Verification items for the finished model (mm, model axes). Face numbers are marked on the shaded views. A direction names the side the tool comes from. Coordinates: 2 decimals unless noted, no trailing zeros. Order: outer loops, then holes, each group sorted by start corner. A loop starts at its lowest first (then second) coordinate and runs counter-clockwise, first axis right, second up. Notation, with made-up numbers: M 31.5,76.5 L 73.5,76.5 A17 cw 73.5,99.5 Z; hole C -2,47.5 d9. An arc over 180 degrees is marked long. Return JSON: item names as keys, results as strings. Group by question number.
Q1. Access from +Z, -Z, +X, -X, +Y, -Y to the whole of each face (thin tool, end or side, straight path). Record for the marked faces 4, 5 and 6.
Q2. Section check A-A, the plane z = 43.5. Enter the section's corners in (x, y).
Q3. Mould release check, pull along X, two halves, no side actions. Record for the marked faces 1, 2 and 3: pulls with the +X half, pulls with the -X half, needs draft (parallel to the pull), parting line crosses it, or undercut.
Q4. Thickness scan on probe 1 along X at (y, z) = (16.25, 8); probe 2 along X at (y, z) = (5, -51.5); probe 3 along Z at (x, y) = (-12, 2.5). Record the ranges inside material, lowest first.
Q5. Go/stop test with flat-tipped pins: pin 1 Ø10 at (x, y) = (4.5, 8.5) entering from -Z; pin 2 Ø10 at (y, z) = (22.5, 5) entering from -X; pin 3 Ø0.8 at (x, y) = (-26, 11) entering from +Z; pin 4 Ø1.5 at (x, z) = (-14.5, -54.5) entering from +Y. Record where each tip stops, or that it passes through.
from build123d import *

# Parameters (mm, degrees)
SKETCH2_W                                       = 55
SKETCH2_H                                       = 135
BOSS_EXTRUDE1_DEPTH                             = 27
SKETCH3_W                                       = 40
SKETCH3_H                                       = 120
CUT_EXTRUDE1_DEPTH                              = 23
SKETCH19_W                                      = 12
SKETCH19_H                                      = 10
CUT_EXTRUDE7_DEPTH                              = 55
SKETCH20_R                                      = 1.25
SKETCH20_W                                      = 9.5
SKETCH20_H                                      = 76
CUT_EXTRUDE8_DEPTH                              = 6
CHAMFER1_SIZE                                   = 10
SKETCH22_R                                      = 0.75
CUT_EXTRUDE10_DEPTH                             = 10
SKETCH23_W                                      = 21.5
SKETCH23_H                                      = 21.5
CUT_EXTRUDE11_DEPTH                             = 1.5
SKETCH24_W                                      = 16
SKETCH24_H                                      = 24
BOSS_EXTRUDE2_DEPTH                             = 7
SKETCH26_W                                      = 11
SKETCH26_H                                      = 4.5
CUT_EXTRUDE13_DEPTH                             = 24
SKETCH27_W                                      = 14.142135623
SKETCH27_H                                      = 3.5
BOSS_EXTRUDE3_DEPTH                             = 8
SKETCH31_W                                      = 29
SKETCH31_H                                      = 10
CUT_EXTRUDE17_DEPTH                             = 3
SKETCH32_W                                      = 8.142135623
SKETCH32_H                                      = 10
CUT_EXTRUDE18_DEPTH                             = 3
MIRROR8_COPY_1_SKETCH_W                         = 8.142135623
MIRROR8_COPY_1_SKETCH_H                         = 10
MIRROR8_COPY_1_DEPTH                            = 3
CSK_FOR_M3_FLAT_HEAD_MACHINE_SCREW2_D           = 3.2
CSK_FOR_M3_FLAT_HEAD_MACHINE_SCREW2_CSINK_D     = 6.3
CSK_FOR_M3_FLAT_HEAD_MACHINE_SCREW2_CSINK_ANGLE = 90
FILLET3_R                                       = 4
MIRROR14_COPY_1_SKETCH_W                        = 14.142135623
MIRROR14_COPY_1_SKETCH_H                        = 3.5
MIRROR14_COPY_1_DEPTH                           = 8
FILLET3_OF_MIRROR14_R                           = 4
FILLET4_R                                       = 4
CSK_FOR_M3_FLAT_HEAD_MACHINE_SCREW3_D           = 3.2
CSK_FOR_M3_FLAT_HEAD_MACHINE_SCREW3_CSINK_D     = 6.3
CSK_FOR_M3_FLAT_HEAD_MACHINE_SCREW3_CSINK_ANGLE = 90
SKETCH46_W                                      = 5.75
SKETCH46_H                                      = 23.5
CUT_EXTRUDE20_DEPTH                             = 2.5


with BuildPart() as part:
    # Sketch2 → Boss-Extrude1 (new body)
    with BuildSketch(Plane(origin=(0, 0, 0), x_dir=(1, 0, 0), z_dir=(0, 1, 0))):
        Rectangle(SKETCH2_W, SKETCH2_H)
    extrude(amount=BOSS_EXTRUDE1_DEPTH)

    # Sketch3 → Cut-Extrude1 (cut)
    with BuildSketch(Plane.XZ):
        Rectangle(SKETCH3_W, SKETCH3_H)
    extrude(amount=-CUT_EXTRUDE1_DEPTH, mode=Mode.SUBTRACT)

    # Sketch19 → Cut-Extrude7 (cut)
    with BuildSketch(Plane(origin=(27.5, 0, 0), x_dir=(0, 0, -1), z_dir=(1, 0, 0))):
        with Locations((-32, 16)):
            Rectangle(SKETCH19_W, SKETCH19_H)
        with Locations((-16, 16)):
            Rectangle(SKETCH19_W, SKETCH19_H)
        with Locations((0, 16)):
            Rectangle(SKETCH19_W, SKETCH19_H)
        with Locations((16, 16)):
            Rectangle(SKETCH19_W, SKETCH19_H)
        with Locations((32, 16)):
            Rectangle(SKETCH19_W, SKETCH19_H)
    extrude(amount=-CUT_EXTRUDE7_DEPTH, mode=Mode.SUBTRACT)

    # Sketch20 → Cut-Extrude8 (cut)
    with BuildSketch(Plane(origin=(0, 27, 0), x_dir=(1, 0, 0), z_dir=(0, 1, 0))):
        with Locations(Location((-14.5, 54.5, 0), (0, 0, 270))):
            Circle(SKETCH20_R)
        with Locations(Location((14.5, 54.5, 0), (0, 0, 270))):
            Circle(SKETCH20_R)
        with Locations(Location((14.5, -54.5, 0), (0, 0, 270))):
            Circle(SKETCH20_R)
        with Locations(Location((-14.5, -54.5, 0), (0, 0, 270))):
            Circle(SKETCH20_R)
        with Locations((-16.75, 10.5)):
            Rectangle(SKETCH20_W, SKETCH20_H)
        with Locations((16.75, 10.5)):
            Rectangle(SKETCH20_W, SKETCH20_H)
    extrude(amount=-CUT_EXTRUDE8_DEPTH, mode=Mode.SUBTRACT)

    # Chamfer1
    chamfer1_edges = [part.edges().sort_by_distance(p)[0] for p in [
        (-27.5, 13.5, -67.5),
        (27.5, 13.5, -67.5),
        (27.5, 13.5, 67.5),
        (-27.5, 13.5, 67.5),
    ]]
    chamfer(chamfer1_edges, length=CHAMFER1_SIZE)

    # Sketch22 → Cut-Extrude10 (cut)
    with BuildSketch(Plane(origin=(0, 27, 0), x_dir=(1, 0, 0), z_dir=(0, 1, 0))):
        with Locations(Location((6, 51.5, 0), (0, 0, 270))):
            Circle(SKETCH22_R)
        with Locations(Location((6, 27.9, 0), (0, 0, 270))):
            Circle(SKETCH22_R)
    extrude(amount=-CUT_EXTRUDE10_DEPTH, mode=Mode.SUBTRACT)

    # Sketch23 → Cut-Extrude11 (cut)
    with BuildSketch(Plane(origin=(0, 27, 0), x_dir=(1, 0, 0), z_dir=(0, 1, 0))):
        with Locations((0, -39.75)):
            Rectangle(SKETCH23_W, SKETCH23_H)
    extrude(amount=-CUT_EXTRUDE11_DEPTH, mode=Mode.SUBTRACT)

    # Sketch24 → Boss-Extrude2 (add)
    with BuildSketch(Plane.XZ.offset(-23)):
        with Locations((0, 13)):
            Rectangle(SKETCH24_W, SKETCH24_H)
    extrude(amount=BOSS_EXTRUDE2_DEPTH)

    # Sketch26 → Cut-Extrude13 (cut)
    with BuildSketch(Plane.XY.offset(25)):
        with Locations((0, 20.75)):
            Rectangle(SKETCH26_W, SKETCH26_H)
    extrude(amount=-CUT_EXTRUDE13_DEPTH, mode=Mode.SUBTRACT)

    # Sketch27 → Boss-Extrude3 (add)
    with BuildSketch(Plane(origin=(-42.5, 0, 42.5), x_dir=(0.7071067811865465, 0, 0.7071067811865487), z_dir=(-0.7071067811865487, 0, 0.7071067811865465))):
        with Locations((28.284271248, 1.75)):
            Rectangle(SKETCH27_W, SKETCH27_H)
    boss_extrude3 = extrude(amount=BOSS_EXTRUDE3_DEPTH)

    # Mirror1: Boss-Extrude3 across plane
    add(boss_extrude3.mirror(Plane(origin=(0, 0, 0), x_dir=(0, 0, 1), z_dir=(1, 0, 0))))

    # Sketch31 → Cut-Extrude17 (cut)
    with BuildSketch(Plane.XY.offset(67.5)):
        with Locations((0, 22)):
            Rectangle(SKETCH31_W, SKETCH31_H)
    cut_extrude17 = extrude(amount=-CUT_EXTRUDE17_DEPTH, mode=Mode.SUBTRACT)

    # Sketch32 → Cut-Extrude18 (cut)
    with BuildSketch(Plane(origin=(42.5, 0, 42.5), x_dir=(0.7071067811865495, 0, -0.7071067811865456), z_dir=(0.7071067811865456, 0, 0.7071067811865495))):
        with Locations((-28.284271248, 22)):
            Rectangle(SKETCH32_W, SKETCH32_H)
    cut_extrude18 = extrude(amount=-CUT_EXTRUDE18_DEPTH, mode=Mode.SUBTRACT)

    # Mirror7: Cut-Extrude18 across plane
    add(cut_extrude18.mirror(Plane(origin=(0, 0, 0), x_dir=(0, 0, 1), z_dir=(1, 0, 0))), mode=Mode.SUBTRACT)

    # Mirror8: Cut-Extrude18 across plane
    add(cut_extrude18.mirror(Plane.XY), mode=Mode.SUBTRACT)

    # Mirror8 copy 1 sketch → Mirror8 copy 1 (cut)
    with BuildSketch(Plane(origin=(-42.5, 0, -42.5), x_dir=(-0.7071067811865495, 0, 0.7071067811865456), z_dir=(-0.7071067811865456, 0, -0.7071067811865495))):
        with Locations((-28.284271248, 22)):
            Rectangle(MIRROR8_COPY_1_SKETCH_W, MIRROR8_COPY_1_SKETCH_H)
    extrude(amount=-MIRROR8_COPY_1_DEPTH, mode=Mode.SUBTRACT)

    # Mirror9: Cut-Extrude17 across plane
    add(cut_extrude17.mirror(Plane.XY), mode=Mode.SUBTRACT)

    # CSK for M3 Flat Head Machine Screw2 (through all)
    with Locations(Plane(origin=(25.329182182, 3.5, 65.327672068), x_dir=(1, 0, 0), z_dir=(0, 1, 0))):
        with Locations((0, 0)):
            CounterSinkHole(CSK_FOR_M3_FLAT_HEAD_MACHINE_SCREW2_D / 2, CSK_FOR_M3_FLAT_HEAD_MACHINE_SCREW2_CSINK_D / 2, counter_sink_angle=CSK_FOR_M3_FLAT_HEAD_MACHINE_SCREW2_CSINK_ANGLE)

    # Fillet3
    fillet3_edges = [part.edges().sort_by_distance(p)[0] for p in [
        (33.156854249, 1.75, 63.156854249),
        (23.156854249, 1.75, 73.156854249),
    ]]
    fillet(fillet3_edges, radius=FILLET3_R)

    # Mirror14: Boss-Extrude3 across plane
    add(boss_extrude3.mirror(Plane.XY))

    # Mirror14 copy 1 sketch → Mirror14 copy 1 (add)
    with BuildSketch(Plane(origin=(42.5, 0, -42.5), x_dir=(-0.7071067811865465, 0, -0.7071067811865487), z_dir=(0.7071067811865487, 0, -0.7071067811865465))):
        with Locations((28.284271248, 1.75)):
            Rectangle(MIRROR14_COPY_1_SKETCH_W, MIRROR14_COPY_1_SKETCH_H)
    extrude(amount=MIRROR14_COPY_1_DEPTH)

    # Fillet3 of Mirror14
    fillet3_of_mirror14_edges = [part.edges().sort_by_distance(p)[0] for p in [
        (33.156854249, 1.75, -63.156854249),
        (23.156854249, 1.75, -73.156854249),
    ]]
    fillet(fillet3_of_mirror14_edges, radius=FILLET3_OF_MIRROR14_R)

    # Fillet4
    fillet4_edges = [part.edges().sort_by_distance(p)[0] for p in [
        (-33.156854249, 1.75, 63.156854249),
        (-23.156854249, 1.75, 73.156854249),
        (-33.156854249, 1.75, -63.156854249),
        (-23.156854249, 1.75, -73.156854249),
    ]]
    fillet(fillet4_edges, radius=FILLET4_R)

    # CSK for M3 Flat Head Machine Screw3 (through all)
    with Locations(Plane(origin=(-25.327672068, 3.5, 65.329182182), x_dir=(1, 0, 0), z_dir=(0, 1, 0))):
        with Locations((0, 0), (-0.001510114, 130.65685425), (50.65685425, 130.65685425)):
            CounterSinkHole(CSK_FOR_M3_FLAT_HEAD_MACHINE_SCREW3_D / 2, CSK_FOR_M3_FLAT_HEAD_MACHINE_SCREW3_CSINK_D / 2, counter_sink_angle=CSK_FOR_M3_FLAT_HEAD_MACHINE_SCREW3_CSINK_ANGLE)

    # Sketch46 → Cut-Extrude20 (cut)
    with BuildSketch(Plane(origin=(27.5, 0, 0), x_dir=(0, 0, -1), z_dir=(1, 0, 0))):
        with Locations((-51.625, 15.25)):
            Rectangle(SKETCH46_W, SKETCH46_H)
        with Locations((-43.875, 15.25)):
            Rectangle(SKETCH46_W, SKETCH46_H)
        with Locations((43.875, 15.25)):
            Rectangle(SKETCH46_W, SKETCH46_H)
        with Locations((51.625, 15.25)):
            Rectangle(SKETCH46_W, SKETCH46_H)
    cut_extrude20 = extrude(amount=-CUT_EXTRUDE20_DEPTH, mode=Mode.SUBTRACT)

    # Mirror15: Cut-Extrude20 across plane
    add(cut_extrude20.mirror(Plane(origin=(0, 0, 0), x_dir=(0, 0, 1), z_dir=(1, 0, 0))), mode=Mode.SUBTRACT)


solid = part.part
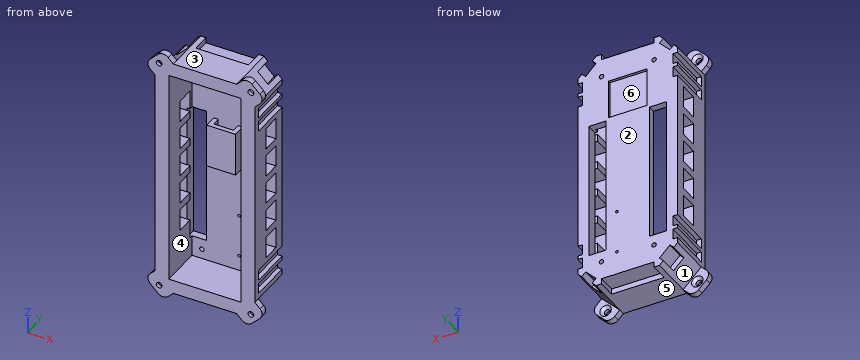
Numbers:
{
 "1": {"face 4": "-Y", "face 5": "-Z, +Y, -Y", "face 6": "+Y"},
 "2": {"outline": "M -27.5,0 L -20,0 L -20,23 L 20,23 L 20,0 L 27.5,0 L 27.5,3.5 L 25,3.5 L 25,27 L 10.75,27 L 10.75,25.5 L -10.75,25.5 L -10.75,27 L -25,27 L -25,3.5 L -27.5,3.5 Z"},
 "3": {"face 1": "pulls with the -X half", "face 2": "needs draft", "face 3": "undercut"},
 "4": {"probe 1": "x = -27.5 to -20, -8 to 8, 20 to 27.5", "probe 2": "x = -25 to -20, 20 to 25", "probe 3": "z = -67.5 to -60, 60 to 67.5"},
 "5": {"pin 1": "stops at z = -67.5", "pin 2": "stops at x = -27.5", "pin 3": "stops at z = 59.4", "pin 4": "passes through"}
}
